Source: three-view drawing plus pictorial views. Frame: mm from the lowest corner of the part. A direction names the side the tool comes from. Coordinates: 2 decimals unless noted, no trailing zeros. Order: outer loops, then holes, each group sorted by start corner. A loop starts at its lowest first (then second) coordinate and runs counter-clockwise, first axis right, second up. Notation, with made-up numbers: (-6.5, 42.5) -> (25.5, 42.5) arc R10 cw to (25.5, 55.5) -> close; hole circle Ø8 at (30, 75). An arc over 180 degrees is marked (long way). Use CSV: the item, a comma, the result in double quotes. Start each with the question number.
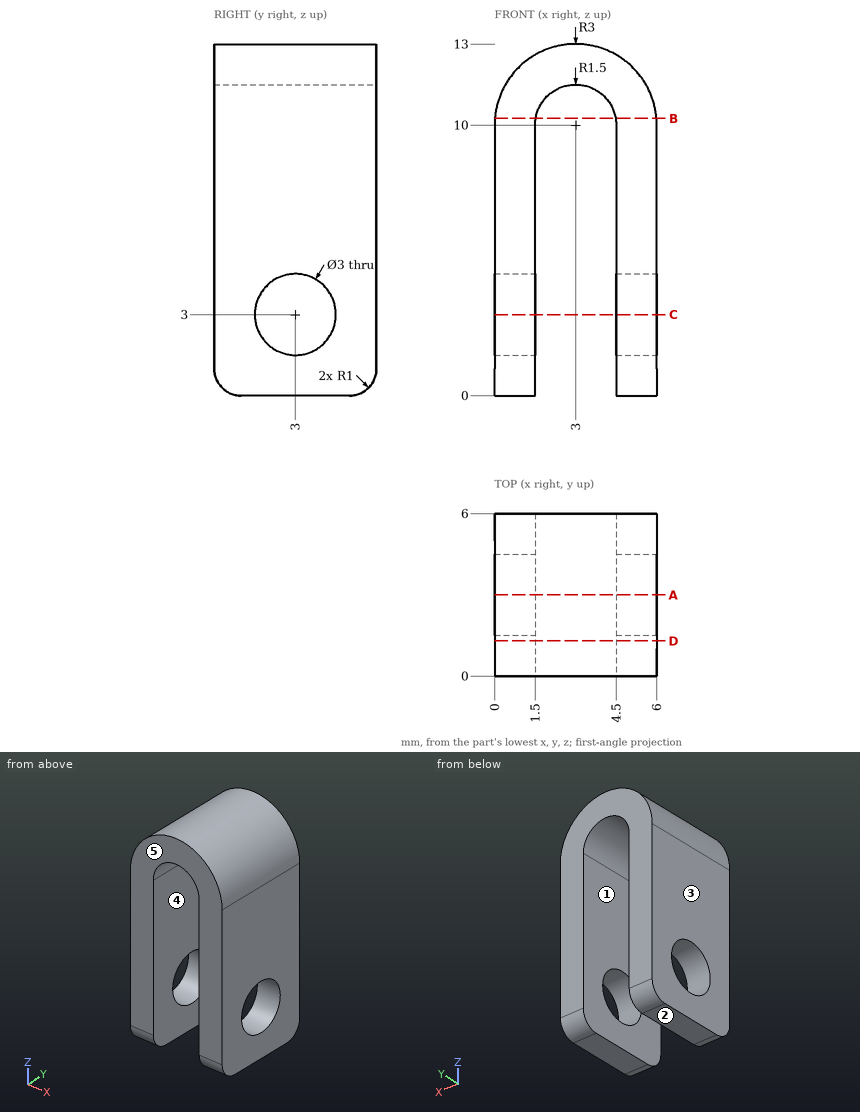
1. Section C-C on z = 3. Return loops of the section in (x, y).
2. Section B-B on z = 10.25. Return loops of the section in (x, y).
3. Material intervals for line 1 along X through (y, z) = (1.4, 5.5); line 2 along Z through (x, y) = (5.6, 3); line 3 along Z through (x, y) = (0.3, 3), sorted ascending.
4. Access query for the marked faces 4 and 5. Directions: +Z, -Z, +X, -X, +Y, -Y. A direction counts if a zero-diameter tool reaches every point of the face in a straight line with its end or side. Return the directions, or none.
5. Contact query for a flat-ended pin moving along its axis: P1, Ø1.8, axis at y = 4.5, z = 4.5, coming from the -X side. Output: stop coordinate, or through.
6. Section D-D on y = 1.3. Return loops of the section in (x, z).
7. Pull-direction query (X, two-part tool) for the marked faces 1, 2 and 3; classes: released by +X, released by -X, zero draft, split by the parting line, or undercut.
8. Section A-A on y = 3. Return loops of the section in (x, z).
Values follow:
1,outline,"(0, 0) -> (1.5, 0) -> (1.5, 1.5) -> (0, 1.5) -> close; (0, 4.5) -> (1.5, 4.5) -> (1.5, 6) -> (0, 6) -> close; (4.5, 0) -> (6, 0) -> (6, 1.5) -> (4.5, 1.5) -> close; (4.5, 4.5) -> (6, 4.5) -> (6, 6) -> (4.5, 6) -> close"
2,outline,"(0.01, 0) -> (1.52, 0) -> (1.52, 6) -> (0.01, 6) -> close; (4.48, 0) -> (5.99, 0) -> (5.99, 6) -> (4.48, 6) -> close"
3,line 1,"x = 0 to 1.5, 4.5 to 6"
3,line 2,"z = 0 to 1.5, 4.5 to 11.5"
3,line 3,"z = 0 to 1.5, 4.5 to 11.31"
4,face 4,"-Z, +Y, -Y"
4,face 5,"+Z, -Z, +X, -X, -Y"
5,P1,"stops at x = 0"
6,outline,"(0, 0) -> (1.5, 0) -> (1.5, 10) arc R1.5 cw to (4.5, 10) -> (4.5, 0) -> (6, 0) -> (6, 10) arc R3 ccw to (0, 10) -> close"
7,face 1,"undercut"
7,face 2,"zero draft"
7,face 3,"released by -X"
8,outline,"(0, 0) -> (1.5, 0) -> (1.5, 1.5) -> (0, 1.5) -> close; (0, 4.5) -> (1.5, 4.5) -> (1.5, 10) arc R1.5 cw to (4.5, 10) -> (4.5, 4.5) -> (6, 4.5) -> (6, 10) arc R3 ccw to (0, 10) -> close; (4.5, 0) -> (6, 0) -> (6, 1.5) -> (4.5, 1.5) -> close"
